from build123d import *

# Parameters (mm, degrees)
SKETCH_1_W          = 160
SKETCH_1_H          = 109
EXTRUDE_1_DEPTH     = 1.6
SKETCH_2_R          = 1.75
CUT_EXTRUDE_1_DEPTH = 2
SKETCH_4_W          = 141
SKETCH_4_H          = 104.7
EXTRUDE_2_DEPTH     = 6
SKETCH_13_W         = 141
SKETCH_13_H         = 2.15
CUT_EXTRUDE_4_DEPTH = 10
CUT_EXTRUDE_2_DEPTH = 1
SKETCH_6_W          = 0.5
SKETCH_6_H          = 0.5
CUT_EXTRUDE_3_DEPTH = 6
EXTRUDE_5_DEPTH     = 3.5
EXTRUDE_6_DEPTH     = 3.5


with BuildPart() as part:
    # 草图1 → 拉伸1 (new body)
    with BuildSketch(Plane.XY):
        Rectangle(SKETCH_1_W, SKETCH_1_H)
    extrude(amount=EXTRUDE_1_DEPTH)

    # 草图2 → 切除-拉伸1 (cut)
    with BuildSketch(Plane(origin=(0, 0, 0), x_dir=(-1, 0, 0), z_dir=(0, 0, -1))):
        with Locations((-76, 50.5)):
            Circle(SKETCH_2_R)
        with Locations((76, 50.5)):
            Circle(SKETCH_2_R)
        with Locations(Location((76, -50.5, 0), (0, 0, 180))):
            Circle(SKETCH_2_R)
        with Locations(Location((-76, -50.5, 0), (0, 0, 180))):
            Circle(SKETCH_2_R)
    extrude(amount=-CUT_EXTRUDE_1_DEPTH, mode=Mode.SUBTRACT)

    # 草图4 → 拉伸2 (add)
    with BuildSketch(Plane(origin=(0, 0, 0), x_dir=(-1, 0, 0), z_dir=(0, 0, -1))):
        with Locations((1.5, 0)):
            Rectangle(SKETCH_4_W, SKETCH_4_H)
    extrude(amount=EXTRUDE_2_DEPTH)

    # 草图13 → 切除-拉伸4 (cut)
    with BuildSketch(Plane(origin=(0, 0, 0), x_dir=(-1, 0, 0), z_dir=(0, 0, -1))):
        with Locations((1.5, 53.425)):
            Rectangle(SKETCH_13_W, SKETCH_13_H)
        with Locations((1.5, -53.425)):
            Rectangle(SKETCH_13_W, SKETCH_13_H)
    extrude(amount=-CUT_EXTRUDE_4_DEPTH, mode=Mode.SUBTRACT)

    # 草图5 → 切除-拉伸2 (cut)
    with BuildSketch(Plane(origin=(0, 0, -6), x_dir=(-1, 0, 0), z_dir=(0, 0, -1))):
        with BuildLine():
            Line((-54.5, 45.95), (66.5, 45.95))
            ThreePointArc((66.5, 45.95), (66.853553391, 45.803553391), (67, 45.45))
            Line((67, 45.45), (67, -45.55))
            ThreePointArc((67, -45.55), (66.853553391, -45.903553391), (66.5, -46.05))
            Line((66.5, -46.05), (-54.5, -46.05))
            ThreePointArc((-54.5, -46.05), (-54.853553391, -45.903553391), (-55, -45.55))
            Line((-55, -45.55), (-55, 45.45))
            ThreePointArc((-55, 45.45), (-54.853553391, 45.803553391), (-54.5, 45.95))
        make_face()
    extrude(amount=-CUT_EXTRUDE_2_DEPTH, mode=Mode.SUBTRACT)

    # 草图6 → 切除-拉伸3 (cut)
    with BuildSketch(Plane(origin=(0, 0, -6), x_dir=(-1, 0, 0), z_dir=(0, 0, -1))):
        with Locations((71.75, 52.1)):
            Rectangle(SKETCH_6_W, SKETCH_6_H)
        with Locations((71.75, -52.1)):
            Rectangle(SKETCH_6_W, SKETCH_6_H)
        with Locations((-68.75, -52.1)):
            Rectangle(SKETCH_6_W, SKETCH_6_H)
        with Locations((-68.75, 52.1)):
            Rectangle(SKETCH_6_W, SKETCH_6_H)
    extrude(amount=-CUT_EXTRUDE_3_DEPTH, mode=Mode.SUBTRACT)

    # 草图10 → 拉伸5 (add)
    with BuildSketch(Plane.XY.offset(1.6)):
        Polygon((67.662920389, -50.358827106), (52.793740241, -50.358827106), (49.146582846, -46.150568574), (50.094290582, -45.280392178), (53.430626839, -49.147509203), (67.662920389, -49.147509203), align=None)
        Polygon((34.038890847, -50.358827106), (19.169710699, -50.358827106), (15.522553304, -46.150568574), (16.470261039, -45.280392178), (19.806597297, -49.147509203), (34.038890847, -49.147509203), align=None)
        Polygon((0.414861305, -50.358827106), (-14.454318843, -50.358827106), (-18.101476238, -46.150568574), (-17.153768503, -45.280392178), (-13.817432245, -49.147509203), (0.414861305, -49.147509203), align=None)
        Polygon((-33.209168237, -50.358827106), (-48.078348385, -50.358827106), (-51.72550578, -46.150568574), (-50.777798045, -45.280392178), (-47.441461787, -49.147509203), (-33.209168237, -49.147509203), align=None)
        Polygon((-50.777798045, 45.280392178), (-51.72550578, 46.150568574), (-48.078348385, 50.358827106), (-33.209168237, 50.358827106), (-33.209168237, 49.147509203), (-47.441461787, 49.147509203), align=None)
        Polygon((-17.153768503, 45.280392178), (-18.101476238, 46.150568574), (-14.454318843, 50.358827106), (0.414861305, 50.358827106), (0.414861305, 49.147509203), (-13.817432245, 49.147509203), align=None)
        Polygon((16.470261039, 45.280392178), (15.522553304, 46.150568574), (19.169710699, 50.358827106), (34.038890847, 50.358827106), (34.038890847, 49.147509203), (19.806597297, 49.147509203), align=None)
        Polygon((67.662920389, 50.358827106), (67.662920389, 49.147509203), (53.430626839, 49.147509203), (50.094290582, 45.280392178), (49.146582846, 46.150568574), (52.793740241, 50.358827106), align=None)
    extrude(amount=EXTRUDE_5_DEPTH)

    # 草图12 → 拉伸6 (add)
    with BuildSketch(Plane(origin=(0, 0, 0), x_dir=(-1, 0, 0), z_dir=(0, 0, -1))):
        Polygon((79.4, 40), (79.4, -40), (72, -45.5), (72, 45.5), align=None)
    extrude(amount=EXTRUDE_6_DEPTH)


solid = part.part
Could you check a few things on this model? Use its own coordinates, in mm. A direction names the side the tool comes from. Round coordinates to 2 decimals unless told otherwise and drop trailing zeros. Write each loop counter-clockwise with the first axis right and the second up, starting at its lowest first coordinate (ties: lowest second). Pieces come first, ordered by that corner, then holes. Notation, with made-up numbers: (-37.75, 46) - (-0.75, 46) arc R25 cw to (-0.75, 63) - close; hole circle Ø6 at (-39.75, -10). An arc over 180 degrees is marked (long way). Put each result on its own line as item: value. Start each with the question number.
(1) Will these pins go through, and if not, where does the flat tip stop? pin 1 (2 mm diameter, centred on x = -76, y = 50.5, fed in from +Z); pin 2 (3 mm diameter, centred on x = 26, z = 4, fed in from +Y); pin 3 (0.6 mm diameter, centred on x = 69, z = -2.5, fed in from +Y); pin 4 (4 mm diameter, centred on x = -10, z = 3.5, fed in from -Y).
(2) Thinking about a two-plate mould opening in X: for faces 1 (the flat face through (-75.648, 42.788, -1.726)), 2 (the flat face through (-15.5, 47.2, 3.3)), 3 (the flat face through (57.8, 49.3, 5.1)), which applies, released by +X, released by -X, zero draft, split by the parting line, or undercut?
(3) I want a section at A-A, the plane x = 76. Please give me the cut outline in (y, z).
(4) I want a section at D-D, the plane x = -44. Please give me the cut outline in (y, z), plus the area to 3 significant figures.
(5) I want a section at B-B, the plane x = -61.5. Please give me the cut outline in (y, z).
(6) For faces 4 (the flat face through (-15.5, -47.2, 3.3)), 5 (the flat face through (27, 50.359, 3)), 6 (the flat face through (-16.3, 48.23, 3.33)), 7 (the flat face through (69, -1, -3)), 8 (the flat face through (-79.4, 1, -2)), which set-ups out of +Z, -Z, +X, -X, +Y, -Y let a thin tool reach every point of the face, with its end or its side?
(7) I want a section at C-C, the plane y = 21. Please give me the cut outline in (x, z).
(8) I need wall thicknesses on probe 1 along Y at (x, z) = (76, 0.5); probe 2 along X at (y, z) = (-50.5, 0.3); probe 3 along Z at (x, y) = (-47, -1). Which ranges of each line are inside material? Lowest first, please.
Here are the results:
1. pin 1: passes through
1. pin 2: stops at y = 50.36
1. pin 3: stops at y = 51.85
1. pin 4: stops at y = -52.35
2. face 1: released by -X
2. face 2: undercut
2. face 3: zero draft
3. outline: (-54.5, 0) - (-52.25, 0) - (-52.25, 1.6) - (-54.5, 1.6) - close; (-48.75, 0) - (48.75, 0) - (48.75, 1.6) - (-48.75, 1.6) - close; (52.25, 0) - (54.5, 0) - (54.5, 1.6) - (52.25, 1.6) - close
4. outline: (-52.35, -6) - (-46.05, -6) - (-46.05, -5) - (45.95, -5) - (45.95, -6) - (52.35, -6) - (52.35, 1.6) - (50.36, 1.6) - (50.36, 5.1) - (49.15, 5.1) - (49.15, 1.6) - (-49.15, 1.6) - (-49.15, 5.1) - (-50.36, 5.1) - (-50.36, 1.6) - (-52.35, 1.6) - close
4. area: 712 mm^2
5. outline: (-52.35, -6) - (-46.05, -6) - (-46.05, -5) - (45.95, -5) - (45.95, -6) - (52.35, -6) - (52.35, 1.6) - (-52.35, 1.6) - close
6. face 4: +Z
6. face 5: +Z, +X, -X, +Y
6. face 6: +Z, +Y
6. face 7: -Z, +X, +Y, -Y
6. face 8: -Z, -X, +Y, -Y
7. outline: (-80, 0) - (-79.4, 0) - (-79.4, -3.5) - (-72, -3.5) - (-72, -6) - (-67, -6) - (-67, -5) - (55, -5) - (55, -6) - (69, -6) - (69, 0) - (80, 0) - (80, 1.6) - (-80, 1.6) - close
8. probe 1: y = -54.5 to -52.25, -48.75 to 48.75, 52.25 to 54.5
8. probe 2: x = -80 to -77.75, -74.25 to 74.25, 77.75 to 80
8. probe 3: z = -5 to 1.6
